For this review, use the dimensioned drawing (mm, ordinates from the lowest corner) and the shaded views. Round coordinates to 2 decimals unless told otherwise and drop trailing zeros. Write each loop counter-clockwise with the first axis right and the second up, starting at its lowest first coordinate (ties: lowest second). Pieces come first, ordered by that corner, then holes.
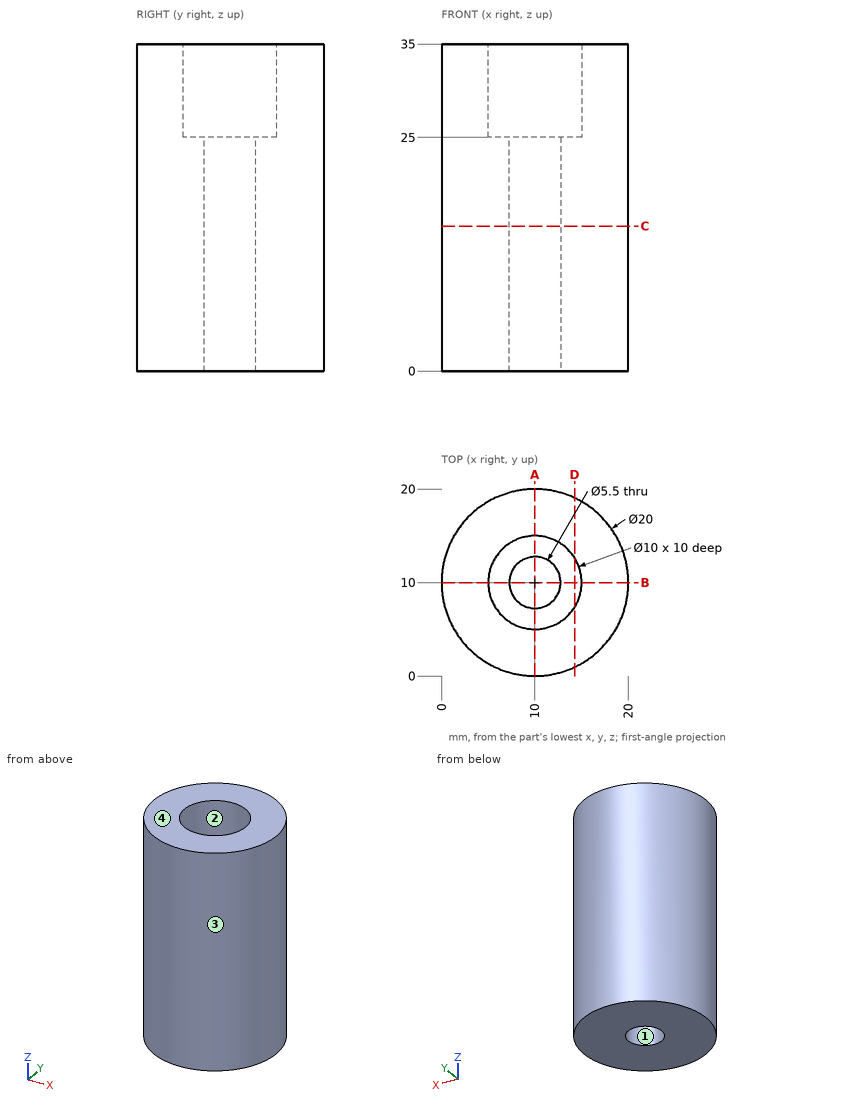
(1) Mouldability with a two-part tool opening along X and no side actions: class the marked faces 1, 2, 3 and 4 as pulls with the +X half, pulls with the -X half, needs draft (parallel to the pull), parting line crosses it, or undercut.
Geometry check:
face 1: undercut
face 2: undercut
face 3: parting line crosses it
face 4: needs draft
(2) We need section A-A, the plane x = 10. Give the boundary of the cut face in (y, z), and give its area (4 significant figures).
Geometry check:
outline: (0, 0) - (7.25, 0) - (7.25, 25) - (5, 25) - (5, 35) - (0, 35) - close; (12.75, 0) - (20, 0) - (20, 35) - (15, 35) - (15, 25) - (12.75, 25) - close
area: 462.5 mm2
(3) For pin 1 Ø1.5 at (x, z) = (13.5, 30.5) entering from +Y; pin 2 Ø1 at (y, z) = (16, 26) entering from -X; pin 3 Ø1.5 at (x, z) = (7.5, 21) entering from -Y; pin 4 Ø12 at (x, z) = (9, 11) entering from +Y, all flat-tipped, find the tip position at first contact; note any pin that passes through.
Geometry check:
pin 1: stops at y = 19.61
pin 2: stops at x = 1.65
pin 3: stops at y = 0.15
pin 4: stops at y = 20
(4) We need section C-C, the plane z = 15.5. Give the boundary of the cut face in (x, y).
Geometry check:
outline: circle Ø20 at (10, 10); hole circle Ø5.5 at (10, 10)
(5) For line 1 along Y through (x, z) = (10, 16.75); line 2 along Y through (x, z) = (10, 32); line 3 along Z through (x, y) = (6.75, 12.25), list the stretches that pass through material, from the lowest coordinate up.
Geometry check:
line 1: y = 0 to 7.25, 12.75 to 20
line 2: y = 0 to 5, 15 to 20
line 3: z = 0 to 25
(6) We need section D-D, the plane x = 14.25. Give the boundary of the cut face in (y, z).
Geometry check:
outline: (0.95, 0) - (19.05, 0) - (19.05, 35) - (12.63, 35) - (12.63, 25) - (7.37, 25) - (7.37, 35) - (0.95, 35) - close
